Input: part model. Units: mm. Frame: model coordinates. Coordinates: 2 decimals unless noted, no trailing zeros. Order: outer loops, then holes, each group sorted by start corner. A loop starts at its lowest first (then second) coordinate and runs counter-clockwise, first axis right, second up. Notation, with made-up numbers: (12.5, 23.25) - (40.5, 23.25) arc R31 cw to (40.5, 52.25) - close; hole circle Ø8 at (-10, 27.25). An arc over 180 degrees is marked (long way). One line per question, with ' | ' between items.
from build123d import *

# Parameters (mm, degrees)
SKETCH_W        = 155
SKETCH_H        = 160
PAD_DEPTH       = 2.5
SKETCH001_W     = 15.25
SKETCH001_H     = 10.25
POCKET_DEPTH    = 2.5
SKETCH002_R     = 2.625
POCKET001_DEPTH = 2.5
POCKET002_DEPTH = 2.5


with BuildPart() as part:
    # Sketch → Pad (new body)
    with BuildSketch(Plane.XY):
        with Locations((0.10674, -30.909095)):
            Rectangle(SKETCH_W, SKETCH_H)
    extrude(amount=PAD_DEPTH)

    # Sketch001 (on Face6 of Pad) → Pocket (cut)
    with BuildSketch(Plane.XY.offset(2.5)):
        with Locations((-64.76826, 38.965905)):
            Rectangle(SKETCH001_W, SKETCH001_H)
        with Locations((-64.76826, -100.784095)):
            Rectangle(SKETCH001_W, SKETCH001_H)
    extrude(amount=-POCKET_DEPTH, mode=Mode.SUBTRACT)

    # Sketch002 (on Face5 of Pocket) → Pocket001 (cut)
    with BuildSketch(Plane.XY.offset(2.5)):
        with Locations((-19.89326, -30.909095)):
            Circle(SKETCH002_R)
        with Locations((-39.89326, -30.909095)):
            Circle(SKETCH002_R)
        with Locations((0.10674, -30.909095)):
            Circle(SKETCH002_R)
        with Locations((20.10674, -30.909095)):
            Circle(SKETCH002_R)
        with Locations((40.10674, -30.909095)):
            Circle(SKETCH002_R)
        with Locations((-39.89326, -10.909095)):
            Circle(SKETCH002_R)
        with Locations((-19.89326, -10.909095)):
            Circle(SKETCH002_R)
        with Locations((0.10674, -10.909095)):
            Circle(SKETCH002_R)
        with Locations((20.10674, -10.909095)):
            Circle(SKETCH002_R)
        with Locations((40.10674, -10.909095)):
            Circle(SKETCH002_R)
        with Locations((-39.89326, -50.909095)):
            Circle(SKETCH002_R)
        with Locations((-19.89326, -50.909095)):
            Circle(SKETCH002_R)
        with Locations((0.10674, -50.909095)):
            Circle(SKETCH002_R)
        with Locations((20.10674, -50.909095)):
            Circle(SKETCH002_R)
        with Locations((40.10674, -50.909095)):
            Circle(SKETCH002_R)
        with Locations((-39.89326, -70.909095)):
            Circle(SKETCH002_R)
        with Locations((-19.89326, -70.909095)):
            Circle(SKETCH002_R)
        with Locations((0.10674, -70.909095)):
            Circle(SKETCH002_R)
        with Locations((20.10674, -70.909095)):
            Circle(SKETCH002_R)
        with Locations((40.10674, -70.909095)):
            Circle(SKETCH002_R)
        with Locations((-39.89326, 9.090905)):
            Circle(SKETCH002_R)
        with Locations((-19.89326, 9.090905)):
            Circle(SKETCH002_R)
        with Locations((0.10674, 9.090905)):
            Circle(SKETCH002_R)
        with Locations((20.10674, 9.090905)):
            Circle(SKETCH002_R)
        with Locations((40.10674, 9.090905)):
            Circle(SKETCH002_R)
    extrude(amount=-POCKET001_DEPTH, mode=Mode.SUBTRACT)

    # Sketch003 (on Face5 of Pocket001) → Pocket002 (cut)
    with BuildSketch(Plane.XY.offset(2.5)):
        Polygon((77.60674, -90.909095), (69.85674, -95.38356), (69.85674, -80.03356), (77.60674, -84.508024), align=None)
        Polygon((77.60674, -34.110166), (69.85674, -38.58463), (69.85674, -23.23463), (77.60674, -27.709095), align=None)
        Polygon((77.60674, 22.689834), (69.85674, 18.21537), (69.85674, 33.56537), (77.60674, 29.090905), align=None)
    extrude(amount=-POCKET002_DEPTH, mode=Mode.SUBTRACT)


solid = part.part
Item 1: Ray query, line 1 (Y direction, x = 20, z = 1.45); line 2 (X direction, y = -32, z = 2.35); line 3 (Y direction, x = 22.5, z = 1.95). Return the intervals inside material, ascending.
Data:
line 1: -110.91 to -73.53, -68.29 to -53.53, -48.29 to -33.53, -28.29 to -13.53, -8.29 to 6.47, 11.71 to 49.09 | line 2: -77.39 to -42.28, -37.51 to -22.28, -17.51 to -2.28, 2.49 to 17.72, 22.49 to 37.72, 42.49 to 69.86 | line 3: -110.91 to -71.99, -69.83 to -51.99, -49.83 to -31.99, -29.83 to -11.99, -9.83 to 8.01, 10.17 to 49.09
Item 2: Contact query for flat-ended pins moving along their axis: P1, Ø3, axis at x = 40.11, y = -30.91, coming from the -Z side; P2, Ø7, axis at x = 40.11, y = -10.91, coming from the +Z side. Output: stop coordinate, or through.
Data:
P1: through | P2: z = 2.5
Item 3: Section B-B on y = -36. Return the cut outline in (x, z), and give its area (3 significant figures).
Data:
outline: (-77.39, 0) - (69.86, 0) - (69.86, 2.5) - (-77.39, 2.5) - close; (74.33, 0) - (77.61, 0) - (77.61, 2.5) - (74.33, 2.5) - close | area: 376 mm^2
Item 4: Section C-C on z = 1.2. Count the separate pieces of the cut face and the enclosed holes in it, and give its area (3 significant figures).
Data:
separate pieces: 1 | enclosed holes: 27 | area: 23,700 mm^2
Item 5: Draft query along X for faces 1 (the face through (73.68, 31.36, 1.27)), 2 (the face through (16, -30, 2.5)). Return one class per face: released by +X, released by -X, zero draft, split by the parting line, or undercut.
Data:
face 1: undercut | face 2: zero draft
Item 6: Section A-A on y = 39. Return the cut outline in (x, z).
Data:
outline: (-77.39, 0) - (-72.39, 0) - (-72.39, 2.5) - (-77.39, 2.5) - close; (-57.14, 0) - (77.61, 0) - (77.61, 2.5) - (-57.14, 2.5) - close
